```python
from build123d import *


with BuildPart() as f1:
    # F0 (on Front) → F1 (revolve)
    with BuildSketch(Plane.XZ):
        Polygon((49.634386, 42.745069), (0, 42.745069), (0, -110.233098), (0, -169.257939), (22.155412, -169.257939), (44.310823, -169.257939), (49.634386, -163.93438), (49.634386, -114.926297), (49.634386, -65.918215), (44.310823, -60.594656), (49.634386, -55.271097), align=None)
        Polygon((0, 110.266026), (0, 42.745069), (49.634386, 42.745069), (12.408596, 110.266026), align=None)
        Polygon((0, 139.329761), (0, 110.266026), (12.408596, 110.266026), (19.418076, 110.266026), (19.418076, 139.329761), align=None)
    revolve(axis=Axis((0, 0, -139.745519), (0, 0, 1)))


solid = f1.part
```
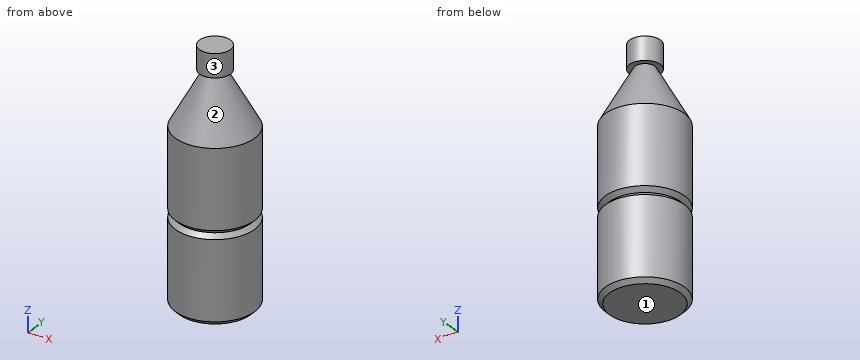
Build history of the part. All positions in model axes, mm. Face numbers are marked on the shaded views. A direction names the side the tool comes from. Round coordinates to 2 decimals unless told otherwise and drop trailing zeros. Write each loop counter-clockwise with the first axis right and the second up, starting at its lowest first coordinate (ties: lowest second). Pieces come first, ordered by that corner, then holes. Notation, with made-up numbers: (57.25, -9.5) - (63.25, -9.5) arc R14 cw to (63.25, 17.5) - close; hole circle Ø7 at (66.25, -13). An arc over 180 degrees is marked (long way). Write each question's results on one line, items separated by ' | '. Start each with the question number.
Item 1: Which spindle directions (+Z, -Z, +X, -X, +Y, -Y) get a long thin tool onto all of the face, cutting with end or side? Do the marked faces 1, 2 and 3. Say none if no direction does.
Item 2: Saw through at B-B (z = -25). Write the cut outline in (x, y), and give its area (3 significant figures).
Item 3: Saw through at A-A (x = 0). Write the cut outline in (y, z).
Item 4: Drop flat-ended pins along their axis: P1, Ø8, axis at x = -29.5, z = -57.5, coming from the -Y side; P2, Ø3, axis at x = -33, y = -37.5, coming from the +Z side; P3, Ø3, axis at x = -22, y = 32.5, coming from the +Z side. Give the stop position or say it passes through.
Item 5: Wall check: L1, parallel to Z at x = -10.5, y = -9.5; L2, parallel to Y at x = -2, z = -20.5; L3, parallel to Z at x = -8.5, y = -13. Give the ranges that are in metal, low to high. Write a range as [from, to].
Item 6: Saw through at D-D (z = 62). Write the cut outline in (x, y).
Results are:
1) face 1: -Z, +X, -X, +Y, -Y | face 2: none | face 3: +Z
2) outline: circle Ø99.27 at (0, 0) | area: 7,740 mm²
3) outline: (-49.63, -163.93) - (-44.31, -169.26) - (44.31, -169.26) - (49.63, -163.93) - (49.63, -65.92) - (44.31, -60.59) - (49.63, -55.27) - (49.63, 42.75) - (12.41, 110.27) - (19.42, 110.27) - (19.42, 139.33) - (-19.42, 139.33) - (-19.42, 110.27) - (-12.41, 110.27) - (-49.63, 42.75) - (-49.63, -55.27) - (-44.31, -60.59) - (-49.63, -65.92) - close
4) P1: stops at y = -42.17 | P2: stops at z = 44.89 | P3: stops at z = 64.31
5) L1: z = [-169.26, 107.09], [110.27, 139.33] | L2: y = [-49.59, 49.59] | L3: z = [-169.26, 104.6], [110.27, 139.33]
6) outline: circle Ø78.04 at (0, 0)
